The model under review builds one solid part; all positions refer to its coordinate system, in mm. Face numbers are marked on the shaded views. A direction names the side the tool comes from. Give positions to 0.01 mm unless a question says otherwise; leave off trailing zeros. Loops run counter-clockwise (first coordinate to the right, second up) from the corner with the lowest first, then second, coordinate; pieces in that order, holes last. Notation, with made-up numbers: M 12,65 L 61,65 A34 cw 61,96 Z; hole C 20.25,72.25 d5. An arc over 180 degrees is marked long. Put each result on its own line as item: value. Start each with the question number.
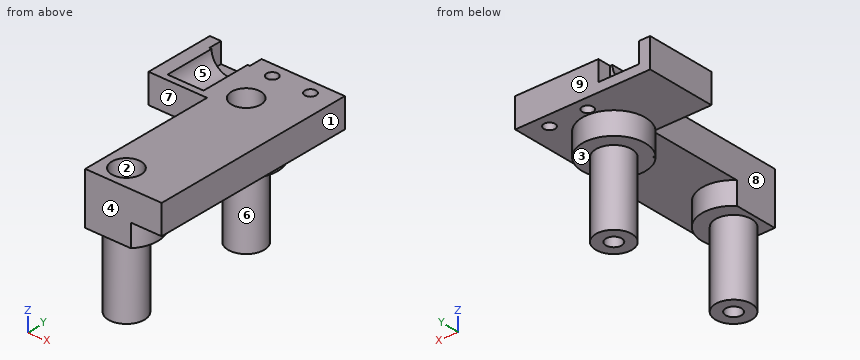
Autodesk Fusion 360 part; units mm, degrees
sketch "Skizze1" plane through (0, 0, 0) normal (0, 0, 1) x (1, 0, 0)
  line L0 (12, -20) -> (-18, -20)
  line L1 (-18, -20) -> (-18, 26.6)
  line L2 (-18, 26.6) -> (12, 26.6)
  line L3 (12, 26.6) -> (12, -20)
  line L4 (-36.0472, 15.24) -> (32.5304, 15.24) construction
  line L5 (-35.3146, -15.24) -> (27.6948, -15.24) construction
  circle A0 centre (0, 15.24) radius 4
  circle A1 centre (0, -15.24) radius 4
  line L6 (-5, -20) -> (-5, 11)
  line L7 (-5, 11) -> (-18, 11)
  circle A2 centre (0, 15.24) radius 7
  circle A3 centre (0, -15.24) radius 7
  line L8 (0, 19) -> (0, -24.3873) construction
  point P0 (0, 15.24)
  point P1 (0, -15.24)
  dimension "d3" = 20
  dimension "d4" = 26.6
  dimension "d5" = 12
  dimension "d6" = 18
  dimension "d7" = 15.24
  dimension "d8" = 15.24
  dimension "d9" = 8
  dimension "d10" = 8
  dimension "d45" = 13
  dimension "d46" = 31
  dimension "d47" = 14
  dimension "d48" = 14
extrude "Extrusion1" add sketch "Skizze1" along normal blind 6.5 contours L0 L1 L2 L3 L6 L7 A2 A3 | L0 L6 A3 | L6 L7 A2 | A0 | A1 picked at (-4.6667, -15.1937) picked at (-3.9058, 10.9235)
sketch "Skizze2" plane through (0, 26.6, 0) normal (0, 1, 0) x (-1, 0, 0)
  line L0 (-12, 0) -> (18, 0)
  line L1 (18, 0) -> (18, 6.5)
  line L2 (18, 6.5) -> (-12, 6.5)
  line L3 (-12, 6.5) -> (-12, 0)
  line L4 (11, 13.5) -> (11, -12.5) construction
  line L5 (6.5, 6.5) -> (15.5, 6.5)
  line L6 (15.5, 6.5) -> (15.5, 2)
  line L7 (15.5, 2) -> (6.5, 2)
  line L8 (6.5, 2) -> (6.5, 6.5)
  line L9 (7, 8.5) -> (7, -2.5) construction
  line L10 (15, 8.4924) -> (15, -3.3602) construction
  arc A0 (7, 6.5) -> (15, 6.5) centre (11, 6.5) ccw
  point P0 (7, 6.5)
  point P1 (7, 6.5)
  point P2 (11, 6.5)
  dimension "d13" = 7
  dimension "d14" = 4.5
  dimension "d15" = 4.5
  dimension "d16" = 4.5
  dimension "d17" = 4
  dimension "d18" = 4
extrude "Extrusion2" cut sketch "Skizze2" against normal blind 3 contours L2 L5 L6 L7 L8 A0
extrude "Extrusion3" cut sketch "Skizze2" against normal blind 14.2 contours L2 L5 A0
extrude "Extrusion6" add sketch "Skizze1" against normal blind 5 contours L0 L6 A3 picked at (-4.6667, -15.1937)
extrude "Extrusion7" add sketch "Skizze1" against normal blind 5 contours L6 L7 A2 picked at (-3.9058, 10.9235)
extrude "Extrusion4" add sketch "Skizze1" against normal blind 21.5 contours A0 | A1
sketch "Skizze3" plane through (0, 0, -21.5) normal (0, 0, -1) x (1, 0, 0)
  circle A0 centre (0, -15.24) radius 4
  line L0 (0, -27) -> (0, 23.61) construction
  line L1 (21.7334, -15.24) -> (-22.4317, -15.24) construction
  line L2 (22.3444, 15.24) -> (-24, 15.24) construction
  point P0 (0, -15.24)
  point P1 (0, 15.24)
  dimension "d25" = 15.24
  dimension "d26" = 15.24
hole "Bohrung1" at (0, 15.24, -21.5) at (0, -15.24, -21.5) direction (0, 0, 1) diameter 3.5 depth 30 tip angle 180
sketch "Skizze6" plane through (0, 0, 6.5) normal (0, 0, 1) x (-1, 0, 0)
  line L0 (15, -12.4) -> (15, -23.6)
  line L1 (15, -23.6) -> (15.5, -23.6)
  line L2 (15.5, -23.6) -> (15.5, -26.6)
  line L3 (15.5, -26.6) -> (18, -26.6)
  line L4 (18, -26.6) -> (18, -11)
  line L5 (18, -11) -> (5, -11)
  line L6 (5, -11) -> (5, 20)
  line L7 (5, 20) -> (-12, 20)
  line L8 (-12, 20) -> (-12, -26.6)
  line L9 (-12, -26.6) -> (6.5, -26.6)
  line L10 (6.5, -26.6) -> (6.5, -23.6)
  line L11 (6.5, -23.6) -> (7, -23.6)
  line L12 (7, -23.6) -> (7, -12.4)
  line L13 (7, -12.4) -> (15, -12.4)
  line L14 (22.7431, -15.24) -> (-23, -15.24) construction
  line L15 (16, 15.24) -> (-23, 15.24) construction
  line L16 (0, -29.9031) -> (0, 26.376) construction
  circle A0 centre (0, -15.24) radius 1.75
  circle A1 centre (0, 15.24) radius 1.75
  point P0 (0, -15.24)
  point P1 (0, 15.24)
  dimension "d53" = 15.24
  dimension "d54" = 15.24
hole "Bohrung3" at (0, 15.24, 6.5) at (0, -15.24, 6.5) direction (0, 0, -1) diameter 6.5 depth 6.5 tip angle 90
sketch "Skizze4" plane through (0, 0, 6.5) normal (0, 0, 1) x (-1, 0, 0)
  line L0 (15, -12.4) -> (15, -23.6)
  line L1 (15, -23.6) -> (15.5, -23.6)
  line L2 (15.5, -23.6) -> (15.5, -26.6)
  line L3 (15.5, -26.6) -> (18, -26.6)
  line L4 (18, -26.6) -> (18, -11)
  line L5 (5, 20) -> (-12, 20)
  line L6 (-12, 20) -> (-12, -26.6)
  line L7 (-12, -26.6) -> (6.5, -26.6)
  line L8 (6.5, -26.6) -> (6.5, -23.6)
  line L9 (6.5, -23.6) -> (7, -23.6)
  line L10 (7, -23.6) -> (7, -12.4)
  line L11 (7, -12.4) -> (15, -12.4)
  line L12 (-23.7996, -23.6) -> (40, -23.6) construction
  line L13 (-7, -34.5714) -> (-7, -14.6073) construction
  line L14 (1.5, -34.5334) -> (1.5, -15.6973) construction
  line L15 (-12, -26.6) -> (-12, 20)
  line L16 (18, -11) -> (5, -11)
  line L17 (5, -11) -> (5, 20)
  circle A0 centre (0, -15.24) radius 3.25
  circle A1 centre (0, 15.24) radius 3.25
  point P0 (-7, -23.6)
  point P1 (1.5, -23.6)
  dimension "d30" = 3
  dimension "d31" = 5
  dimension "d32" = 5
  dimension "d33" = 8.5
hole "Bohrung2" at (7, 23.6, 6.5) at (-1.5, 23.6, 6.5) direction (0, 0, -1) diameter 2.5 depth 8 tip angle 180
ref_plane "Arbeitsebene1" through (0, 0, 2.7) normal (0, 0, 1) x (1, 0, 0)
sketch "Skizze5" plane through (0, 0, 2.7) normal (0, 0, 1) x (1, 0, 0)
  line L0 (18, 23.6) -> (-21, 23.6) construction
  line L1 (-18, 26.6) -> (12, 26.6)
  line L2 (7, 19.6167) -> (7, 31.5736) construction
  line L3 (-1.5, 19.6924) -> (-1.5, 31.9243) construction
  line L4 (12, 26.6) -> (12, -20)
  line L5 (5.7298, 25.8) -> (4.4597, 23.6)
  line L6 (4.4597, 23.6) -> (5.7298, 21.4)
  line L7 (5.7298, 21.4) -> (8.2702, 21.4)
  line L8 (8.2702, 21.4) -> (9.5403, 23.6)
  line L9 (9.5403, 23.6) -> (8.2702, 25.8)
  line L10 (8.2702, 25.8) -> (5.7298, 25.8)
  line L11 (-2.7702, 25.8) -> (-4.0403, 23.6)
  line L12 (-4.0403, 23.6) -> (-2.7702, 21.4)
  line L13 (-2.7702, 21.4) -> (-0.2298, 21.4)
  line L14 (-0.2298, 21.4) -> (1.0403, 23.6)
  line L15 (1.0403, 23.6) -> (-0.2298, 25.8)
  line L16 (-0.2298, 25.8) -> (-2.7702, 25.8)
  point P0 (7, 23.6)
  point P1 (-1.5, 23.6)
  dimension "d38" = 3
  dimension "d39" = 5
  dimension "d40" = 8.5
  dimension "d41" = 4.4
  dimension "d42" = 4.4
extrude "Extrusion5" cut sketch "Skizze5" along normal blind 1.8
(1) For the marked faces 1, 2, 3, 4 and 5, list the 3-axis set-ups (+Z, -Z, +X, -X, +Y, -Y) from which the entire face can be reached by the end or side of a thin tool; tool diameter is ignored.
(2) We need section B-B, the plane z = -18.5. Write out the cut boundary in (x, y), plus the area to 3 significant figures.
(3) We need section C-C, the plane x = -11. Write out the cut boundary in (y, z).
(4) We need section D-D, the plane z = 1. Write out the cut boundary in (x, y).
(5) We need section A-A, the plane y = -15.24. Write out the cut boundary in (x, z).
(6) Draft analysis for pull direction Y (two halves, no side actions). For the marked faces 6, 7, 8 and 9, state which applies: +Y half, -Y half, draft (parallel to the pull), parting line (faces both ways), or undercut.
(7) Insertion check: pin 1 (2 mm diameter, centred on x = -9, z = 5.5, fed in from +Y); pin 2 (4 mm diameter, centred on y = 22, z = -6.5, fed in from +X); pin 3 (3 mm diameter, centred on y = 18.5, z = -7.5, fed in from -X). Each pin has a flat end and moves straight along its axis. Give the tip position at first contact, or say it passes through.
(8) To check wall thickness, follow L1, parallel to Y at x = 0, z = -13; L2, parallel to Y at x = 7, z = 5.7; L3, parallel to Z at x = 8.25, y = 22. State the ranges of each line that lie inside material, in increasing order. Write a range as [from, to].
Check sheet entries:
1. face 1: +Z, -Z, +X, +Y, -Y
1. face 2: +Z
1. face 3: -Z
1. face 4: +Z, -Z, +X, -X, -Y
1. face 5: +Z, +Y
2. outline: C 0,-15.24 d8; C 0,15.24 d8; hole C 0,-15.24 d3.5; hole C 0,15.24 d3.5
2. area: 81.3 mm²
3. outline: M 11,0 L 26.6,0 L 26.6,2 L 23.6,2 L 23.6,2.5 L 12.4,2.5 L 12.4,6.5 L 11,6.5 Z
4. outline: M -18,11 L -5,11 L -5,-20 L 12,-20 L 12,26.6 L -18,26.6 Z; hole C 0,-15.24 d6.5; hole C 0,15.24 d6.5; hole C -1.5,23.6 d2.5; hole C 7,23.6 d2.5
5. outline: M -5,-5 L -4,-5 L -4,-21.5 L -1.75,-21.5 L -1.75,-1.5 L -3.25,0 L -3.25,6.5 L -5,6.5 Z; M 1.75,-21.5 L 4,-21.5 L 4,-5 L 7,-5 L 7,0 L 12,0 L 12,6.5 L 3.25,6.5 L 3.25,0 L 1.75,-1.5 Z
6. face 6: undercut
6. face 7: -Y half
6. face 8: draft
6. face 9: +Y half
7. pin 1: stops at y = 12.4
7. pin 2: stops at x = 4.41
7. pin 3: stops at x = -3.59
8. L1: y = [-19.24, -16.99], [-13.49, -11.24], [11.24, 13.49], [16.99, 19.24]
8. L2: y = [-20, 22.35], [24.85, 26.6]
8. L3: z = [0, 2.7], [4.5, 6.5]
